Autodesk Inventor part; units mm, degrees
ref_plane "Work Plane1" through (0, -12.3, 0) normal (0, -1, 0) x (1, 0, 0)
ref_plane "YZ Plane" through (0, 0, 0) normal (1, 0, 0) x (0, 1, 0)
ref_plane "XZ Plane" through (0, 0, 0) normal (0, 1, 0) x (-1, 0, 0)
sketch "Sketch1" plane through (0, 0, 0) normal (0, 1, 0) x (-1, 0, 0)
  circle A0 centre (0, 0) radius 5
  dimension "d0" = 10
extrude "Extrusion1" add sketch "Sketch1" along normal blind 9.5
sketch "Sketch2" plane through (0, 9.5, 0) normal (0, 1, 0) x (1, 0, 0)
  circle A0 centre (0, 0) radius 3.5
  dimension "d3" = 7
extrude "Extrusion2" add sketch "Sketch2" along normal blind 2.3
sketch "Sketch3" plane through (0, 0, 0) normal (0, -1, 0) x (1, 0, 0)
  line L0 (5.4, -5.4) -> (-5.4, -5.4)
  line L1 (-5.4, -5.4) -> (-5.4, 5.4)
  line L2 (-5.4, 5.4) -> (5.4, 5.4)
  line L3 (5.4, 5.4) -> (5.4, -5.4)
  line L4 (5.4, -5.4) -> (-5.4, 5.4) construction
  line L5 (-5.4, -5.4) -> (5.4, 5.4) construction
  point P0 (0, 0)
  dimension "d6" = 10.8
  dimension "d7" = 10.8
ref_plane "Work Plane1" through (0, -12.3, 0) normal (0, -1, 0) x (1, 0, 0)
sketch "Sketch4" plane through (0, -12.3, 0) normal (0, -1, 0) x (1, 0, 0)
  line L0 (6.9, -6) -> (-6.9, -6)
  line L1 (-6.9, -6) -> (-6.9, 6)
  line L2 (-6.9, 6) -> (6.9, 6)
  line L3 (6.9, 6) -> (6.9, -6)
  line L4 (6.9, -6) -> (-6.9, 6) construction
  line L5 (-6.9, -6) -> (6.9, 6) construction
  point P0 (0, 0)
  dimension "d9" = 13.8
  dimension "d10" = 12
loft "Loft1" add profiles "Sketch3", "Sketch4"
sketch "Sketch6" plane through (-6.9, -12.3, -6) normal (0, -1, 0) x (1, 0, 0)
  line L0 (12.3, 0.6) -> (13.8, 0)
  line L1 (0, 12) -> (13.8, 12)
  line L2 (13.8, 12) -> (13.8, 0)
  line L3 (13.8, 0) -> (0, 0)
  line L4 (0, 0) -> (0, 12)
  line L5 (0, 12) -> (13.8, 0) construction
  line L6 (13.8, 12) -> (0, 0) construction
  point P0 (6.9, 6)
extrude "Extrusion3" add sketch "Sketch6" along normal blind 9
fillet "Fillet2" radius 1 8 edges at (6.15, -6.15, -5.7) (-6.15, -6.15, -5.7) (6.15, -6.15, 5.7) (-6.15, -6.15, 5.7) (6.9, -16.8, 6) (6.9, -16.8, -6) (-6.9, -16.8, 6) (-6.9, -16.8, -6)
sketch "Sketch8" plane through (-6.9, -21.3, -6) normal (0, -1, 0) x (1, 0, 0)
  line L0 (1.0015, 12) -> (12.7985, 12)
  line L1 (11.9, 12) -> (11.9, 2)
  line L2 (11.9, 2) -> (1.9, 2)
  line L3 (1.9, 2) -> (1.9, 12)
  line L4 (1.9, 12) -> (11.9, 12)
  line L5 (13.8, 1) -> (13.8, 11)
  line L6 (0, 11) -> (0, 1)
  point P0 (6.9, 6)
  dimension "d25" = 10
  dimension "d26" = 10
  dimension "d27" = 1.9
  dimension "d29" = 1.9
extrude "Extrusion5" add sketch "Sketch8" along normal blind 4
sketch "Sketch9" plane through (0, 11.8, 0) normal (0, 1, 0) x (1, 0, 0)
  circle A0 centre (0, 0) radius 1.175
  circle A1 centre (0, 0) radius 2.75
  dimension "d32" = 2.35
  dimension "d33" = 5.5
extrude "Extrusion6" cut sketch "Sketch9" against normal blind 7.9
fillet "Fillet3" radius 0.5 1 edges at (-1.175, 11.8, 0)
fillet "Fillet4" radius 0.3 1 edges at (-3.5, 11.8, 0)
fillet "Fillet5" radius 0.3 1 edges at (-2.75, 11.8, 0)
properties part number "ConectorFuente"
Verification items for the finished model (mm, model axes). A direction names the side the tool comes from. Coordinates: 2 decimals unless noted, no trailing zeros.
1. Scan lines: line 1 (Z direction, x = 0, y = 6.5) (3 decimals); line 2 (X direction, y = 8, z = 1); line 3 (Y direction, x = -0.25, z = -4.75). Record each from-to range of solid material in increasing order.
Results found:
line 1: z = -5 to -2.75, -1.175 to 1.175, 2.75 to 5
line 2: x = -4.9 to -2.56, -0.62 to 0.62, 2.56 to 4.9
line 3: y = -21.3 to 9.5
2. Set-up check for faces 1 (the face through (0, -23, -4)), 2 (the face through (6.615, -16.731, -5.699)), 3 (the face through (5, -23, 1)), 4 (the face through (1.08, 4.68, 4.88)): record each of +Z, -Z, +X, -X, +Y, -Y from which the full face is reachable in a straight line by a thin tool's end or side.
Results found:
face 1: -Z, +X, -X, -Y
face 2: -Z, +X, +Y, -Y
face 3: +Z, -Z, +X, -Y
face 4: +Y
3. Go/stop test with flat-tipped pins: pin 1 Ø4.5 at (y, z) = (-24, 1.5) entering from -X; pin 2 Ø3 at (x, y) = (-1, -23.5) entering from -Z; pin 3 Ø8 at (x, y) = (0, -0.5) entering from +Z. Record where each tip stops, or that it passes through.
Results found:
pin 1: stops at x = -5
pin 2: stops at z = -4
pin 3: stops at z = 5.62
